For this review, take the finished solid that the model builds, in its own axes (mm). Coordinates: 2 decimals unless noted, no trailing zeros. Loops run counter-clockwise (first coordinate to the right, second up) from the corner with the lowest first, then second, coordinate; pieces in that order, holes last.
1. To check wall thickness, follow probe 1 along X at (y, z) = (14, 3.3); probe 2 along X at (y, z) = (36, 2.8); probe 3 along X at (y, z) = (30.5, 1.8). State the ranges of each line that lie inside material, in increasing order.
2. Take a section at C-C, the plane z = 4.95. Count the separate pieces of the cut face and the enclosed holes in it, then the cut area to 3 significant figures.
3. Clearance check with flat-ended pins moving along their axes: P1, Ø3, axis at y = 1.5, z = 4, coming from the +X side; P2, Ø2.5, axis at y = 36.5, z = 3, coming from the -X side; P3, Ø1.8, axis at x = 64, z = 3.5, coming from the +Y side. State where each tip first meets the part, or that it passes through.
4. Take a section at A-A, the plane y = 21. State the section outline as (x, z) points, then the cut area to 3 significant figures.
5. Take a section at D-D, the plane x = 98. State the section outline as (y, z) points.
6. Take a section at B-B, the plane x = 210. State the section outline as (y, z) points.
```python
from build123d import *

# Parameters (mm, degrees)
SKETCH_2_W      = 6
SKETCH_2_H      = 6
EXTRUDE_1_DEPTH = 6


with BuildPart() as part:
    # Эскиз2 → Бобышка-Вытянуть1 (new body)
    with BuildSketch(Plane.XY):
        Polygon((89, 38), (89, 8), (109, 8), (109, 38), (129, 38), (129, 35), (166.5, 35), (166.5, 38), (186.5, 38), (186.5, 35), (224, 35), (224, 38), (244, 38), (244, 30), (250, 30), (250, 24), (244, 24), (244, 16), (250, 16), (250, 10), (244, 10), (244, 0), (177, 0), (177, 6), (172, 6), (172, 0), (0, 0), (0, 10), (-6, 10), (-6, 16), (0, 16), (0, 24), (-6, 24), (-6, 30), (0, 30), (0, 38), (20, 38), (20, 35), (34.5, 35), (34.5, 38), (54.5, 38), (54.5, 35), (69, 35), (69, 38), align=None)
        with Locations((78, 27)):
            Rectangle(SKETCH_2_W, SKETCH_2_H, mode=Mode.SUBTRACT)
        with Locations((78, 13)):
            Rectangle(SKETCH_2_W, SKETCH_2_H, mode=Mode.SUBTRACT)
    extrude(amount=EXTRUDE_1_DEPTH)


solid = part.part
```
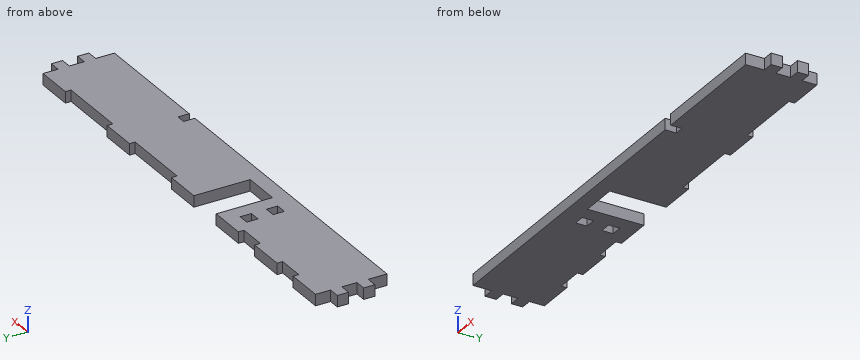
Results list:
1. probe 1: x = -6 to 75, 81 to 89, 109 to 250
1. probe 2: x = 0 to 20, 34.5 to 54.5, 69 to 89, 109 to 129, 166.5 to 186.5, 224 to 244
1. probe 3: x = 0 to 89, 109 to 244
2. separate pieces: 1
2. enclosed holes: 2
2. area: 8,400 mm2
3. P1: stops at x = 244
3. P2: stops at x = 0
3. P3: stops at y = 35
4. outline: (0, 0) - (89, 0) - (89, 6) - (0, 6) - close; (109, 0) - (244, 0) - (244, 6) - (109, 6) - close
4. area: 1,340 mm2
5. outline: (0, 0) - (8, 0) - (8, 6) - (0, 6) - close
6. outline: (0, 0) - (35, 0) - (35, 6) - (0, 6) - close
